Source: CAD feature listing. Evaluate the final solid. Frame: model axes, mm. Give positions to 0.01 mm unless a question says otherwise; leave off trailing zeros. Order: outer loops, then holes, each group sorted by start corner. A loop starts at its lowest first (then second) coordinate and runs counter-clockwise, first axis right, second up.
1) Section C-C, the plane x = 2.2. Give the number of separate pieces and of enclosed holes in the cut face, plus the area to 3 significant figures.
2) Section D-D, the plane y = 71. Return loops of the section in (x, z), plus the area to 3 significant figures.
3) Draft query along Z for faces 1 (the face through (2, -67, 546)), 2 (the face through (2.46, -559.21, 660.47)), 3 (the face through (5, -263, 69)). Return one class per face: released by +Z, released by -Z, zero draft, split by the parting line, or undercut.
4) First-contact query: P1, Ø19, axis at y = 38.77, z = 361.99, coming from the -X side; P2, Ø2, axis at x = 4, z = 541.5, coming from the -Y side; P3, Ø2, axis at x = 2.5, z = 200.5, coming from the +Y side. Flat tips, straight axial feed; report the tip coordinate or a pass-through.
5) Section B-B, the plane z = 425.5. Return loops of the section in (x, y).
6) Section A-A, the plane y = -76.5. Return loops of the section in (x, z), plus the area to 3 significant figures.
7) Material intervals for line 1 (Y direction, x = 4.7, z = 503); line 2 (Z direction, x = 0.3, y = -103.5); line 3 (Y direction, x = 3.65, z = 454), sorted ascending.
```python
from build123d import *

# Parameters (mm, degrees)
SKETCH1_R           = 250
BOSS_EXTRUDE1_DEPTH = 5
SKETCH2_R           = 6
CUT_EXTRUDE1_DEPTH  = 10
CIRPATTERN1_COUNT   = 12


with BuildPart() as part:
    # Sketch1 → Boss-Extrude1 (new body)
    with BuildSketch(Plane(origin=(0, 0, 0), x_dir=(0, 0, -1), z_dir=(1, 0, 0))):
        with BuildLine():
            Line((-126.985698369, 168.770507744), (193.014301631, 168.770507744))
            Line((193.014301631, 168.770507744), (193.014301631, -166.625210225))
            ThreePointArc((193.014301631, -166.625210225), (29.499330124, -553.664543235), (-361.985698369, -706.229492256))
            ThreePointArc((-361.985698369, -706.229492256), (-663.674001264, -555.574607548), (-771.985698369, -236.229492256))
            ThreePointArc((-771.985698369, -236.229492256), (-634.689640971, 20.877775707), (-361.985698369, 123.770507744))
            Line((-361.985698369, 123.770507744), (-126.985698369, 123.770507744))
            Line((-126.985698369, 123.770507744), (-126.985698369, 168.770507744))
        make_face()
        with Locations((-361.985698369, -236.229492256)):
            Circle(SKETCH1_R, mode=Mode.SUBTRACT)
    extrude(amount=BOSS_EXTRUDE1_DEPTH)

    # Sketch2 → Cut-Extrude1 (cut)
    with BuildSketch(Plane(origin=(5, 0, 0), x_dir=(0, 0, -1), z_dir=(1, 0, 0))):
        with Locations((-86.985698369, -236.229492256)):
            Circle(SKETCH2_R)
    cut_extrude1 = extrude(amount=-CUT_EXTRUDE1_DEPTH, mode=Mode.SUBTRACT)

    # CirPattern1: Cut-Extrude1 ×12 about axis
    cirpattern1_axis = Axis((0, -236.229492256, 361.985698369), (1, 0, 0))
    for i in range(1, CIRPATTERN1_COUNT):
        add(cut_extrude1.rotate(cirpattern1_axis, i * 360 / CIRPATTERN1_COUNT), mode=Mode.SUBTRACT)


solid = part.part
```
From the geometry:
1. separate pieces: 1
1. enclosed holes: 13
1. area: 479,000 mm2
2. outline: (0, -193.01) - (5, -193.01) - (5, 563.81) - (0, 563.81) - close
2. area: 3,780 mm2
3. face 1: undercut
3. face 2: released by +Z
3. face 3: zero draft
4. P1: stops at x = 0
4. P2: stops at y = -654.08
4. P3: stops at y = 123.77
5. outline: (0, -696.93) - (5, -696.93) - (5, -478.03) - (0, -478.03) - close; (0, 5.57) - (5, 5.57) - (5, 118.8) - (0, 118.8) - close
6. outline: (0, -193.01) - (5, -193.01) - (5, 169.67) - (0, 169.67) - close; (0, 554.3) - (5, 554.3) - (5, 716.1) - (0, 716.1) - close
6. area: 2,620 mm2
7. line 1: y = -672.13 to -479.25, -469.52 to -442.66, -29.8 to -2.94, 6.79 to 98.86
7. line 2: z = -193.01 to 120.19, 127.47 to 150.13, 573.84 to 596.5, 603.78 to 731.03
7. line 3: y = -689.63 to -468.68, -3.78 to 113.32
